Autodesk Inventor part; units mm, degrees
ref_plane "YZ Plane" through (0, 0, 0) normal (1, 0, 0) x (0, 1, 0)
ref_plane "XZ Plane" through (0, 0, 0) normal (0, 1, 0) x (-1, 0, 0)
ref_plane "XY Plane" through (0, 0, 0) normal (0, 0, 1) x (1, 0, 0)
sketch "Skizze1" plane through (0, 0, 0) normal (1, 0, 0) x (0, 1, 0)
  line L0 (-28, 0) -> (28, 0) construction
  line L1 (0, 35) -> (0, -35) construction
  line L2 (-20, -25) -> (20, -25)
  line L3 (20, -25) -> (20, 25)
  line L4 (20, 25) -> (-20, 25)
  line L5 (-20, 25) -> (-20, -25)
  line L6 (-20, -25) -> (20, 25) construction
  line L7 (20, -25) -> (-20, 25) construction
  point P0 (0, 0)
  dimension "d0" = 40
  dimension "d1" = 50
extrude "Grundkörper" add sketch "Skizze1" along normal mid plane 20
sketch "Skizze2" plane through (10, 0, 0) normal (1, 0, 0) x (0, 0, -1)
  line L0 (-25, 20) -> (-25, -20) construction
  line L1 (0, -28) -> (0, 28) construction
  line L2 (-35, 0) -> (35, 0) construction
  line L3 (-25, -10) -> (5, -10)
  line L4 (5, -10) -> (5, 10)
  line L5 (5, 10) -> (-25, 10)
  line L6 (-25, 10) -> (-25, -10)
  line L7 (25, -20) -> (25, 20) construction
  line L8 (25, -8.4) -> (20, -8.4)
  line L9 (12, -0.4) -> (12, 0.4)
  line L10 (20, 8.4) -> (25, 8.4)
  line L11 (25, -8.4) -> (25, 8.4)
  arc A0 (12, -0.4) -> (20, -8.4) centre (20, -0.4) ccw
  arc A1 (20, 8.4) -> (12, 0.4) centre (20, 0.4) ccw
  point P0 (0, 0)
  dimension "d4" = 30
  dimension "d5" = 20
  dimension "d14" = 13
  dimension "d15" = 16.8
  dimension "d16" = 8
extrude "Ausschnitt" cut sketch "Skizze2" against normal through all
sketch "Skizze4" plane through (-10, -20, -25) normal (0, -1, 0) x (1, 0, 0)
  line L0 (20, 20) -> (0, 20) construction
  line L1 (20, 50) -> (0, 50) construction
  line L2 (10, 60) -> (10, -10)
  line L3 (0, 35) -> (20, 35) construction
  line L4 (0, 0) -> (0, 50) construction
  line L5 (20, 50) -> (20, 0) construction
  point P0 (10, 25)
  point P1 (10, 42.5)
  point P2 (10, 27.5)
  dimension "d19" = 30
  dimension "d20" = 15
  dimension "d21" = 15
hole "DIN7984_M5_Boh" at (0, -20, 17.5) at (0, -20, 2.5) direction (0, 1, 0) diameter 5.5 end up to surface counterbore diameter 10 counterbore depth 3.9
mirror "Spiegeln_DIN7984_M5_Boh" about plane through (0, 0, 0) normal (0, 1, 0) of "DIN7984_M5_Boh"
sketch "Skizze5" plane through (10, -20, -25) normal (0, 0, -1) x (-1, 0, 0)
  line L0 (0, 0) -> (20, 0) construction
  line L1 (20, 11.6) -> (0, 11.6) construction
  line L2 (20, 40) -> (0, 40) construction
  line L3 (0, 28.4) -> (20, 28.4) construction
  line L4 (10, -8) -> (10, 48) construction
  line L5 (-4, 20) -> (24, 20) construction
  line L6 (10, 11.6) -> (10, 0) construction
  point P0 (10, 20)
  point P1 (10, 5.8)
  point P2 (10, 34.2)
  dimension "d29" = 28.4
hole "M5x10" at (0, -14.2, -25) at (0, 14.2, -25) direction (0, 0, 1) diameter 4.134 depth 14.2 tip angle 118 countersink diameter 5 countersink angle 90
sketch "Skizze" plane through (10, -20, -25) normal (0, 0, -1) x (-1, 0, 0)
  circle A0 centre (10, 5.8) radius 2.5
  line L0 (20, 11.6) -> (0, 11.6)
  line L1 (0, 0) -> (0, 11.6)
  line L2 (0, 0) -> (20, 0)
  line L3 (20, 11.6) -> (20, 0)
  circle A1 centre (10, 34.2) radius 2.5
  line L4 (0, 28.4) -> (20, 28.4)
  line L5 (20, 40) -> (20, 28.4)
  line L6 (20, 40) -> (0, 40)
  line L7 (0, 28.4) -> (0, 40)
  line L8 (0, 11.6) -> (0, 19.6)
  line L9 (0, 19.6) -> (0, 20.4)
  line L10 (0, 20.4) -> (0, 28.4)
  line L11 (20, 28.4) -> (20, 20.4)
  line L12 (20, 20.4) -> (20, 19.6)
  line L13 (20, 19.6) -> (20, 11.6)
  point P0 (10, 20)
chamfer "Fase_Allgemein" distance 4 angle 45 4 edges at (10, -20, 0) (-10, -20, 0) (10, 20, 0) (-10, 20, 0)
chamfer "Fase" distance 0.5 angle 45 15 edges at (10, -6.0569, -14.3431) (10, 0, -12) (10, 6.0569, -14.3431) (10, 8.4, -22.5) (10, -8.4, -22.5) (-10, 6.0569, -14.3431) (-10, 0, -12) (-10, -6.0569, -14.3431) (-10, -8.4, -22.5) (-10, 8.4, -22.5) (-10, 0, -5) (-10, 10, 10) (10, -10, 10) (10, 0, -5) (10, 10, 10)
equation "\"d20\" = 0.5 * d19"
properties part number "200-50-WHEEL-CONNECTOR-20MM-01" material "Aluminium 6061"
Geometry check sheet. Reference: the model listing, model coordinates, mm. A direction names the side the tool comes from. Coordinates: 2 decimals unless noted, no trailing zeros. Order: outer loops, then holes, each group sorted by start corner. A loop starts at its lowest first (then second) coordinate and runs counter-clockwise, first axis right, second up.
Q1. Sectioned sample at C-C on z = 2.5. Give the number of separate pieces and of enclosed holes in the cut face, and give its area (3 significant figures).
Reply:
separate pieces: 4
enclosed holes: 0
area: 223 mm2
Q2. Sectioned sample at A-A on z = 10. Record the cut outline in (x, y).
Reply:
outline: (-10, -16) - (-6, -20) - (6, -20) - (10, -16) - (10, -10.5) - (9.5, -10) - (-10, -10) - close; (-10, 10.5) - (-9.5, 10) - (9.5, 10) - (10, 10.5) - (10, 16) - (6, 20) - (-6, 20) - (-10, 16) - close
Q3. Thickness scan on probe 1 along Z at (x, y) = (0, 18.95); probe 2 along Y at (x, z) = (5.25, 0.5); probe 3 along X at (y, z) = (11.25, 2.5). Record the ranges inside material, lowest first.
Reply:
probe 1: z = -25 to -2.5, 7.5 to 12.5, 22.5 to 25
probe 2: y = -20 to -10, 10 to 20
probe 3: x = -10 to -2.75, 2.75 to 10
Q4. Tool access check on faces 1 (the face through (1.05, 13.01, 5.04)), 2 (the face through (-0.22, 18.023, 12.505)), 3 (the face through (2, -16.1, 15)), 4 (the face through (0, -15, 25)), 5 (the face through (0, 8.4, -22)). Record the directions out of +Z, -Z, +X, -X, +Y, -Y that give a thin tool (end or side, any length) a straight path to the whole face; none if there is none.
Reply:
face 1: +Y, -Y
face 2: +Y
face 3: -Y
face 4: +Z, +X, -X, +Y, -Y
face 5: -Z, +X, -X
Q5. Depth check by flat-ended pin: pin 1 Ø1.5 at (x, z) = (-7, -15.5) entering from +Y; pin 2 Ø6.5 at (x, z) = (0, 17.5) entering from -Y; pin 3 Ø9 at (x, z) = (0, 2.5) entering from +Y. Enter the tip coordinate at first touch or a pass-through.
Reply:
pin 1: stops at y = 19.75
pin 2: stops at y = -16.1
pin 3: stops at y = 16.1
Q6. Sectioned sample at B-B on x = -7. Record the cut outline in (y, z), and give its area (3 significant figures).
Reply:
outline: (-19, -25) - (-8.4, -25) - (-8.4, -20) arc R8 cw to (-0.4, -12) - (0.4, -12) arc R8 cw to (8.4, -20) - (8.4, -25) - (19, -25) - (19, 25) - (10, 25) - (10, -5) - (-10, -5) - (-10, 25) - (-19, 25) - close
area: 1,110 mm2
Q7. Draft check along X on faces 6 (the face through (0, -10, 10)), 7 (the face through (-8, -18, 0)), 8 (the face through (0, -14.6, -9.8)). Enter one of: released by +X, released by -X, zero draft, split by the parting line, or undercut.
Reply:
face 6: zero draft
face 7: released by -X
face 8: undercut
